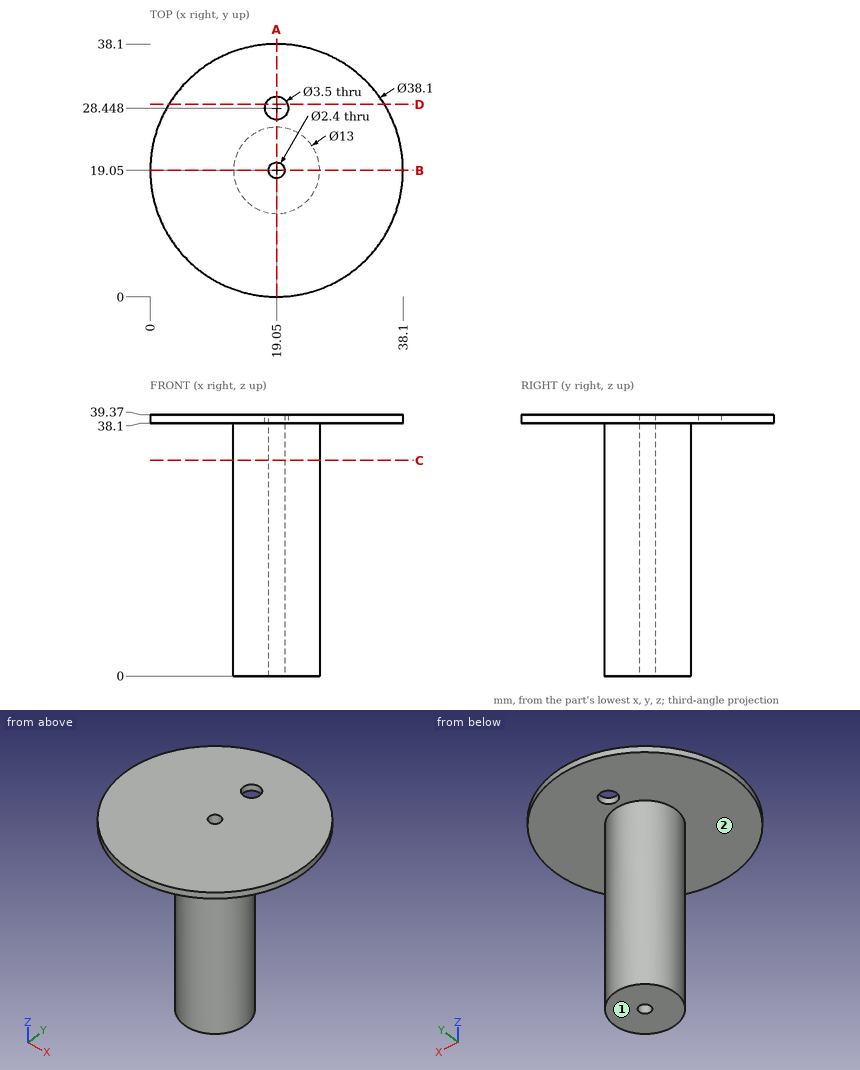
Verification items for this drawing (mm, ordinates from the low corner). A direction names the side the tool comes from. Coordinates: 2 decimals unless noted, no trailing zeros. Loops run counter-clockwise (first coordinate to the right, second up) from the corner with the lowest first, then second, coordinate; pieces in that order, holes last. Notation, with made-up numbers: (-32.75, 42.25) - (23.25, 42.25) arc R27 ccw to (23.25, 65.25) - close; hole circle Ø3 at (29.25, 22.5). An arc over 180 degrees is marked (long way). One line per item, written item: value. Start each with the question number.
(1) Cross-section at B-B on y = 19.05. Enter the section's corners in (x, z).
(2) Cross-section at D-D on y = 29. Enter the section's corners in (x, z) (3 decimals), plus the area to 3 significant figures.
(3) Tool access check on the marked faces 1 and 2. Record the directions out of +Z, -Z, +X, -X, +Y, -Y that give a thin tool (end or side, any length) a straight path to the whole face; none if there is none.
(4) Cross-section at C-C on z = 32.5. Enter the section's corners in (x, y), plus the area to 3 significant figures.
(5) Depth check by flat-ended pin: P1, Ø2, axis at y = 13.5, z = 16, coming from the -X side; P2, Ø8, axis at y = 25, z = 31, coming from the +X side; P3, Ø12, axis at y = 24, z = 24.5, coming from the +X side; P4, Ø5, axis at y = 30, z = 25.5, coming from the -X side. Enter the tip coordinate at first touch or a pass-through.
(6) Material ranges on line 1 (Y direction, x = 19.05, z = 38.75); line 2 (Y direction, x = 19, z = 38), recorded low to high. Write a range as [from, to].
(7) Cross-section at A-A on x = 19.05. Enter the section's corners in (y, z).
Results below:
1. outline: (0, 38.1) - (12.55, 38.1) - (12.55, 0) - (17.85, 0) - (17.85, 39.37) - (0, 39.37) - close; (20.25, 0) - (25.55, 0) - (25.55, 38.1) - (38.1, 38.1) - (38.1, 39.37) - (20.25, 39.37) - close
2. outline: (2.805, 38.1) - (17.389, 38.1) - (17.389, 39.37) - (2.805, 39.37) - close; (20.711, 38.1) - (35.295, 38.1) - (35.295, 39.37) - (20.711, 39.37) - close
2. area: 37.0 mm2
3. face 1: -Z, +X, -X, +Y, -Y
3. face 2: -Z
4. outline: circle Ø13 at (19.05, 19.05); hole circle Ø2.4 at (19.05, 19.05)
4. area: 128 mm2
5. P1: stops at x = 14.41
5. P2: stops at x = 25.25
5. P3: stops at x = 25.55
5. P4: passes through
6. line 1: y = [0, 17.85], [20.25, 26.7], [30.2, 38.1]
6. line 2: y = [12.55, 17.85], [20.25, 25.55]
7. outline: (0, 38.1) - (12.55, 38.1) - (12.55, 0) - (17.85, 0) - (17.85, 39.37) - (0, 39.37) - close; (20.25, 0) - (25.55, 0) - (25.55, 38.1) - (26.7, 38.1) - (26.7, 39.37) - (20.25, 39.37) - close; (30.2, 38.1) - (38.1, 38.1) - (38.1, 39.37) - (30.2, 39.37) - close
